Drawing for the job (mm, zero at the part's lowest x, y, z). A direction names the side the tool comes from. Round coordinates to 2 decimals unless told otherwise and drop trailing zeros. Order: outer loops, then holes, each group sorted by start corner. A loop starts at its lowest first (then second) coordinate and runs counter-clockwise, first axis right, second up. Notation, with made-up numbers: (68, 84) - (115, 84) arc R14 cw to (115, 106) - close; hole circle Ø8 at (5.25, -35). An arc over 180 degrees is marked (long way). Put each result on its own line as item: value. Start each with the question number.
Item 1: Mould opens along Z. For the marked faces 5, 6 and 7 say: pulls with the +Z half, pulls with the -Z half, needs draft (parallel to the pull), parting line crosses it, or undercut.
Item 2: Saw through at D-D on x = 37.5. List the corners of the cut face in (y, z), plus the area to 3 significant figures.
Item 3: Pin check, flat tips, straight feed: pin 1 Ø1.5 at (x, z) = (80, 21.5) entering from +Y; pin 2 Ø12 at (y, z) = (83, 36) entering from +X; pin 3 Ø10 at (x, y) = (150.5, 65.5) entering from -Z; pin 4 Ø12 at (x, y) = (72, 63.5) entering from -Z. Stop position of each tip, or through.
Item 4: Saw through at A-A on z = 8. List the corners of the cut face in (x, y), plus the area to 3 significant figures.
Item 5: Probe probe 1 along Z at (x, y) = (78, 60); probe 2 along Y at (x, z) = (40, 8); probe 3 along Z at (x, y) = (80.5, 77.5). List the from-to ranges inside material, lowest first.
Item 6: Which spindle directions (+Z, -Z, +X, -X, +Y, -Y) get a long thin tool onto all of the face, cutting with end or side? Do the marked faces 1, 2, 3 and 4. Say none if no direction does.
Item 7: Saw through at B-B on y = 58. List the corners of the cut face in (x, z).
Item 8: Saw through at C-C on x = 12. List the corners of the cut face in (y, z).
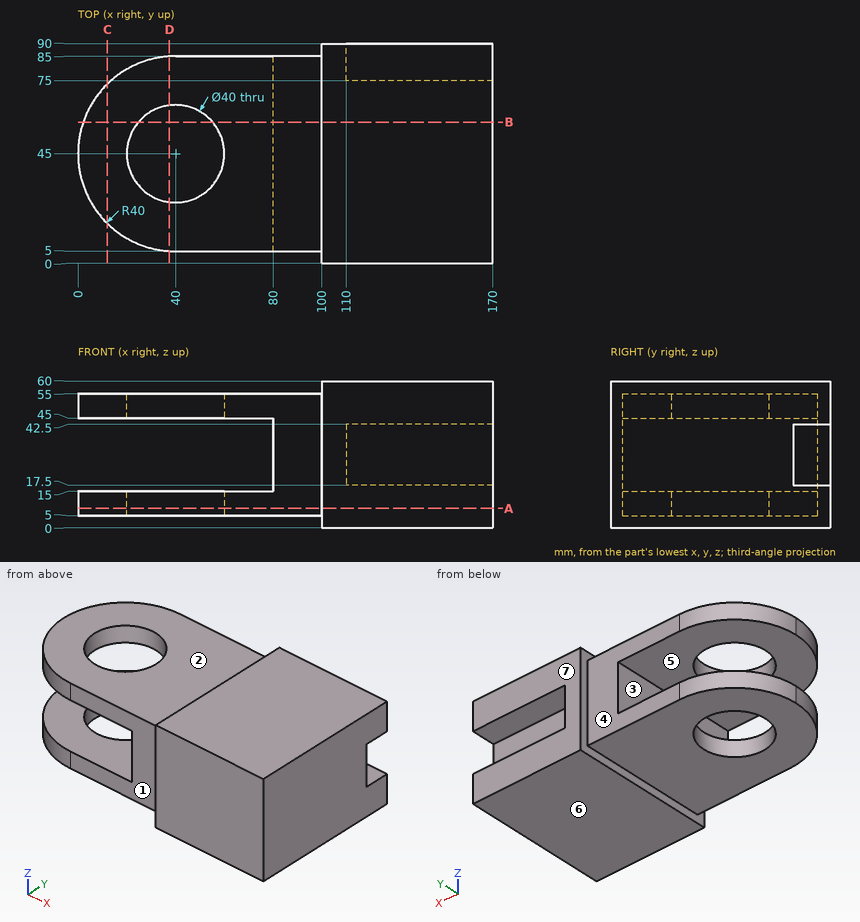
Results found:
1. face 5: undercut
1. face 6: pulls with the -Z half
1. face 7: needs draft
2. outline: (5.08, 5) - (25.16, 5) - (25.16, 15) - (5.08, 15) - close; (5.08, 45) - (25.16, 45) - (25.16, 55) - (5.08, 55) - close; (64.84, 5) - (84.92, 5) - (84.92, 15) - (64.84, 15) - close; (64.84, 45) - (84.92, 45) - (84.92, 55) - (64.84, 55) - close
2. area: 803 mm²
3. pin 1: stops at y = 85
3. pin 2: stops at x = 110
3. pin 3: stops at z = 0
3. pin 4: stops at z = 5
4. outline: (40, 5) - (100, 5) - (100, 0) - (170, 0) - (170, 90) - (100, 90) - (100, 85) - (40, 85) arc R40 ccw to start; hole circle Ø40 at (40, 45)
4. area: 12,400 mm²
5. probe 1: z = 5 to 15, 45 to 55
5. probe 2: y = 5 to 25, 65 to 85
5. probe 3: z = 5 to 55
6. face 1: +Z, -Z, -X, -Y
6. face 2: +Z, -X, +Y, -Y
6. face 3: -X, +Y, -Y
6. face 4: +Z, -Z, -X, +Y
7. outline: (2.17, 5) - (24.8, 5) - (24.8, 15) - (2.17, 15) - close; (2.17, 45) - (24.8, 45) - (24.8, 55) - (2.17, 55) - close; (55.2, 5) - (100, 5) - (100, 0) - (170, 0) - (170, 60) - (100, 60) - (100, 55) - (55.2, 55) - (55.2, 45) - (80, 45) - (80, 15) - (55.2, 15) - close
8. outline: (16.43, 5) - (73.57, 5) - (73.57, 15) - (16.43, 15) - close; (16.43, 45) - (73.57, 45) - (73.57, 55) - (16.43, 55) - close
